Part model, mm, in its own coordinate system. Face numbers are marked on the shaded views. A direction names the side the tool comes from. Round coordinates to 2 decimals unless told otherwise and drop trailing zeros. Write each loop counter-clockwise with the first axis right and the second up, starting at its lowest first coordinate (ties: lowest second). Pieces come first, ordered by that corner, then holes. Notation, with made-up numbers: (53.5, 21.5) -> (64.5, 21.5) arc R9 cw to (64.5, 37.5) -> close; hole circle Ø6 at (40, 62.25). An arc over 180 degrees is marked (long way). Return JSON: item names as keys, results as strings. Group by question number.
(1) Drop flat-ended pins along their axis: pin 1 Ø1 at (y, z) = (1, 1) entering from +X; pin 2 Ø1 at (y, z) = (-2.5, 0) entering from -X. Give the stop position or say it passes through.
(2) Saw through at D-D (y = -2.5). List the corners of the cut face in (x, z), plus the area to 3 significant figures.
(3) Saw through at A-A (x = 0). List the corners of the cut face in (y, z).
(4) Drill centre lines: L1, parallel to Y at x = 1.55, z = -1.35; L2, parallel to X at y = 1, z = -1.6; L3, parallel to Z at x = 0.1, y = 1.75. Where is each one in solid material? Low to high. Write a range as from..to.
(5) Saw through at B-B (z = 0). List the corners of the cut face in (x, y).
(6) Saw through at C-C (y = 2.5). List the corners of the cut face in (x, z).
(7) Tool access for the marked faces 1 and 2: list every direction of +Z, -Z, +X, -X, +Y, -Y with a clear straight run to the whole face (end or side of a thin tool).
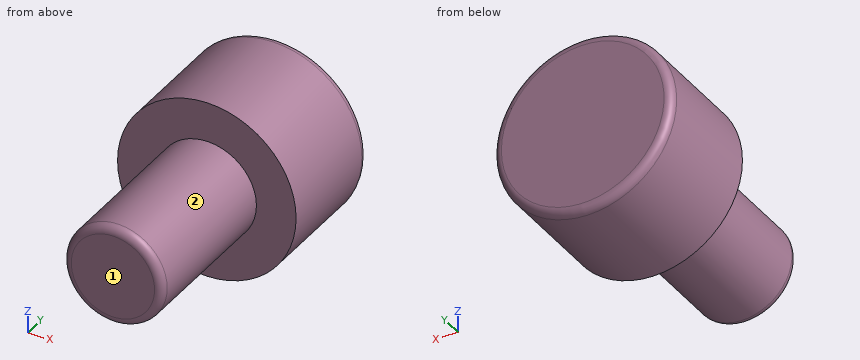
from build123d import *

# Parameters (mm, degrees)
SKETCH1_W   = 2.25
SKETCH1_H   = 3
SKETCH1_W_2 = 1.25
SKETCH1_H_2 = 4
FILLET1_R   = 0.2
FILLET2_R   = 0.2


with BuildPart() as part:
    # Sketch1 → Revolve1 (revolve)
    with BuildSketch(Plane.XY):
        with Locations((1.125, 1.5)):
            Rectangle(SKETCH1_W, SKETCH1_H)
        with Locations((0.625, -2)):
            Rectangle(SKETCH1_W_2, SKETCH1_H_2)
    revolve(axis=Axis((0, 0, 0), (0, -1, 0)))

    # Fillet1
    fillet1_edges = [part.edges().sort_by_distance(p)[0] for p in [
        (-2.25, 3, 0),
    ]]
    fillet(fillet1_edges, radius=FILLET1_R)

    # Fillet2
    fillet2_edges = [part.edges().sort_by_distance(p)[0] for p in [
        (-1.25, -4, 0),
    ]]
    fillet(fillet2_edges, radius=FILLET2_R)


solid = part.part
Computed values:
{
 "1": {"pin 1": "x = 2.19", "pin 2": "x = -1.25"},
 "2": {"outline": "circle Ø2.5 at (0, 0)", "area": "4.91 mm2"},
 "3": {"outline": "(-4, -1.05) arc R0.2 ccw to (-3.8, -1.25) -> (0, -1.25) -> (0, -2.25) -> (2.8, -2.25) arc R0.2 ccw to (3, -2.05) -> (3, 2.05) arc R0.2 ccw to (2.8, 2.25) -> (0, 2.25) -> (0, 1.25) -> (-3.8, 1.25) arc R0.2 ccw to (-4, 1.05) -> close"},
 "4": {"L1": "0..3", "L2": "-1.58..1.58", "L3": "-2.25..2.25"},
 "5": {"outline": "(-2.25, 0) -> (-1.25, 0) -> (-1.25, -3.8) arc R0.2 ccw to (-1.05, -4) -> (1.05, -4) arc R0.2 ccw to (1.25, -3.8) -> (1.25, 0) -> (2.25, 0) -> (2.25, 2.8) arc R0.2 ccw to (2.05, 3) -> (-2.05, 3) arc R0.2 ccw to (-2.25, 2.8) -> close"},
 "6": {"outline": "circle Ø4.5 at (0, 0)"},
 "7": {"face 1": "+Z, -Z, +X, -X, -Y", "face 2": "-Y"}
}
